Verification items for the finished model (mm, model axes). Round coordinates to 2 decimals unless told otherwise and drop trailing zeros. Loops run counter-clockwise (first coordinate to the right, second up) from the corner with the lowest first, then second, coordinate; pieces in that order, holes last. Notation, with made-up numbers: (62.5, 20) - (117.5, 20) arc R10 ccw to (117.5, 32) - close; hole circle Ø5 at (-21, 14.5). An arc over 180 degrees is marked (long way). Use CSV: the item, a comma, the result in double quotes.
```python
from build123d import *

# Parameters (mm, degrees)
PAD_DEPTH    = 1.65
PAD001_DEPTH = 1.524


with BuildPart() as part:
    # Sketch → Pad (new body)
    with BuildSketch(Plane.XY):
        with BuildLine():
            ThreePointArc((-90.17, -36.195), (-88.682102, -39.787102), (-85.09, -41.275))
            Line((85.09, -41.275), (-85.09, -41.275))
            ThreePointArc((85.09, -41.275), (88.682102, -39.787102), (90.17, -36.195))
            Line((90.17, 36.195), (90.17, -36.195))
            ThreePointArc((90.17, 36.195), (88.682102, 39.787102), (85.09, 41.275))
            Line((-85.09, 41.275), (85.09, 41.275))
            ThreePointArc((-85.09, 41.275), (-88.682102, 39.787102), (-90.17, 36.195))
            Line((-90.17, -36.195), (-90.17, 36.195))
        make_face()
        with BuildLine():
            ThreePointArc((-78.8, -23.038), (-78.576815, -23.576815), (-78.038, -23.8))
            Line((78.038, -23.8), (-78.038, -23.8))
            ThreePointArc((78.038, -23.8), (78.576815, -23.576815), (78.8, -23.038))
            Line((78.8, 23.038), (78.8, -23.038))
            ThreePointArc((78.8, 23.038), (78.576815, 23.576815), (78.038, 23.8))
            Line((-78.038, 23.8), (78.038, 23.8))
            ThreePointArc((-78.038, 23.8), (-78.576815, 23.576815), (-78.8, 23.038))
            Line((-78.8, -23.038), (-78.8, 23.038))
        make_face(mode=Mode.SUBTRACT)
    extrude(amount=PAD_DEPTH)

    # Sketch001 (on Face17 of Pad) → Pad001 (join)
    with BuildSketch(Plane(origin=(0, 0, 0), x_dir=(1, 0, 0), z_dir=(0, 0, -1))):
        with BuildLine():
            ThreePointArc((-90.17, -36.195), (-88.682102, -39.787102), (-85.09, -41.275))
            Line((85.09, -41.275), (-85.09, -41.275))
            ThreePointArc((85.09, -41.275), (88.682102, -39.787102), (90.17, -36.195))
            Line((90.17, 36.195), (90.17, -36.195))
            ThreePointArc((90.17, 36.195), (88.682102, 39.787102), (85.09, 41.275))
            Line((-85.09, 41.275), (85.09, 41.275))
            ThreePointArc((-85.09, 41.275), (-88.682102, 39.787102), (-90.17, 36.195))
            Line((-90.17, -36.195), (-90.17, 36.195))
        make_face()
    extrude(amount=PAD001_DEPTH)


solid = part.part
```
1) Cross-section at A-A, the plane z = 1. Record the cut outline in (x, y) (3 decimals), then the cut area to 3 significant figures.
Returned:
outline,"(-90.17, -36.195) arc R5.08 ccw to (-85.09, -41.275) - (85.09, -41.275) arc R5.08 ccw to (90.17, -36.195) - (90.17, 36.195) arc R5.08 ccw to (85.09, 41.275) - (-85.09, 41.275) arc R5.08 ccw to (-90.17, 36.195) - close; hole (-78.8, -23.038) arc R0.762 ccw to (-78.038, -23.8) - (78.038, -23.8) arc R0.762 ccw to (78.8, -23.038) - (78.8, 23.038) arc R0.762 ccw to (78.038, 23.8) - (-78.038, 23.8) arc R0.762 ccw to (-78.8, 23.038) - close"
area,"7,360 mm²"
2) Cross-section at B-B, the plane y = -21. Record the cut outline in (x, z), then the cut area to 3 significant figures.
Returned:
outline,"(-90.17, -1.52) - (90.17, -1.52) - (90.17, 1.65) - (78.8, 1.65) - (78.8, 0) - (-78.8, 0) - (-78.8, 1.65) - (-90.17, 1.65) - close"
area,"312 mm²"
3) Cross-section at C-C, the plane x = -57.5. Record the cut outline in (y, z) (3 decimals).
Returned:
outline,"(-41.275, -1.524) - (41.275, -1.524) - (41.275, 1.65) - (23.8, 1.65) - (23.8, 0) - (-23.8, 0) - (-23.8, 1.65) - (-41.275, 1.65) - close"
4) Mould release check, pull along Y, two halves, no side actions. Record for faces 1 (the face through (88.64, 39.83, 0.09)), 2 (the face through (88.72, -39.75, 0.09)), 3 (the face through (-90.17, 1, 0)), 4 (the face through (-1, 0, 0)): +Y half, -Y half, draft (parallel to the pull), parting line (faces both ways), or undercut.
Returned:
face 1,"+Y half"
face 2,"-Y half"
face 3,"draft"
face 4,"undercut"
5) Thickness scan on probe 1 along Y at (x, z) = (69.5, 0.65) (3 decimals); probe 2 along X at (y, z) = (-8, 0.75); probe 3 along Z at (x, y) = (-18, -9). Record the ranges inside material, lowest first. Write a range as [from, to].
Returned:
probe 1,"y = [-41.275, -23.8], [23.8, 41.275]"
probe 2,"x = [-90.17, -78.8], [78.8, 90.17]"
probe 3,"z = [-1.52, 0]"
6) Gauge pin test, flat end, axial feed: pin 1 Ø8 at (x, y) = (63.5, 7.5) entering from +Z. Record the tip position at first contact, or that the pin passes through.
Returned:
pin 1,"stops at z = 0"
